```python
from build123d import *

# Parameters (mm, degrees)
F1_DEPTH = 77.5
F3_DEPTH = 15
F3_TAPER = -30
F4_W     = 9.7201652825
F4_H     = 81.3968237489
F5_DEPTH = 15


with BuildPart() as f1:
    # F0 (on Front) → F1 (new body, symmetric)
    with BuildSketch(Plane.XZ):
        Polygon((-0.1256162198, -11.1232604972), (9.5702180536, -5.6704170861), (9.6958342734, 5.4528434111), (0.1256162198, 11.1232604972), (-9.5702180536, 5.6704170861), (-9.6958342734, -5.4528434111), align=None)
    extrude(amount=F1_DEPTH, both=True)

    # F2 (on face) → F3 (join)
    with BuildSketch(Plane(origin=(0, 77.5, 0), x_dir=(-1, 0, 0), z_dir=(0, 1, 0))):
        Polygon((0.2229186467, -19.7393472), (17.2062354526, -9.676620389), (16.983316806, 10.062726811), (-0.2229186467, 19.7393472), (-17.2062354526, 9.676620389), (-16.983316806, -10.062726811), align=None)
        Polygon((9.6958342734, -5.4528434111), (0.1256162198, -11.1232604972), (-9.5702180536, -5.6704170861), (-9.6958342734, 5.4528434111), (-0.1256162198, 11.1232604972), (9.5702180536, 5.6704170861), align=None, mode=Mode.SUBTRACT)
        Polygon((-9.5702180536, -5.6704170861), (0.1256162198, -11.1232604972), (9.6958342734, -5.4528434111), (9.5702180536, 5.6704170861), (-0.1256162198, 11.1232604972), (-9.6958342734, 5.4528434111), align=None)
    extrude(amount=F3_DEPTH, taper=F3_TAPER)

    # F4 (on Top) → F5 (join)
    with BuildSketch(Plane.XY):
        with Locations((-0.1620021649, 46.2903873995)):
            Rectangle(F4_W, F4_H)
    extrude(amount=F5_DEPTH)


solid = f1.part
```
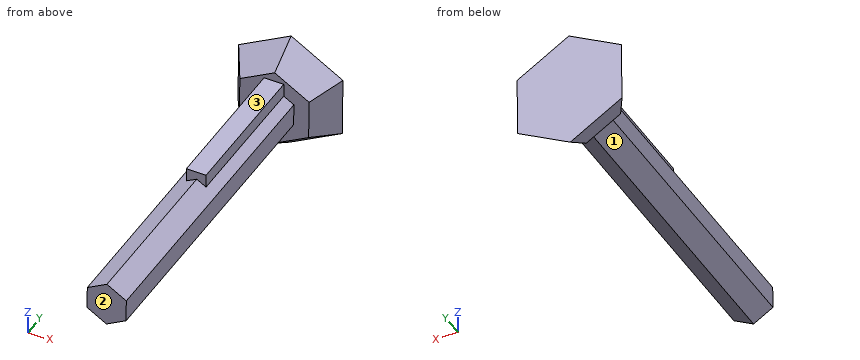
Input: part model. Units: mm. Frame: model coordinates. Face numbers are marked on the shaded views. A direction names the side the tool comes from. Coordinates: 2 decimals unless noted, no trailing zeros. Loops run counter-clockwise (first coordinate to the right, second up) from the corner with the lowest first, then second, coordinate; pieces in that order, holes last. Notation, with made-up numbers: (78, 84) - (91, 84) arc R32 cw to (91, 121) - close; hole circle Ø9 at (-24.75, 51). An arc over 180 degrees is marked (long way). Answer in a Markdown table with one row per item.
(1) Cut plane B-B on y = 2. Output: boundary loops of the cut face in (x, z).
Model answer:
| item | result |
|---|---|
| outline | (-9.7, -5.45) - (-0.13, -11.12) - (9.57, -5.67) - (9.7, 5.45) - (0.13, 11.12) - (-9.57, 5.67) - close |
(2) Material intervals for L1, parallel to Y at x = -1, z = -14.5; L2, parallel to X at y = -32.5, z = -3.5; L3, parallel to Y at x = 23, z = 6.5, sorted ascending. Write a range as from..to.
Model answer:
| item | result |
|---|---|
| L1 | y = 77.5..92.5 |
| L2 | x = -9.67..9.59 |
| L3 | y = 87.6..92.5 |
(3) Pin query (flat end, axial travel): P1, Ø8, axis at x = 1.5, y = 43.5, coming from the +Z side; P2, Ø8, axis at y = -53, z = 16.5, coming from the -X side; P3, Ø7, axis at y = 49, z = 13, coming from the +X side; P4, Ø3, axis at y = 75.5, z = -6, coming from the -X side. Return the tip coordinate at first contact, or that it passes through.
Model answer:
| item | result |
|---|---|
| P1 | stops at z = 15 |
| P2 | passes through |
| P3 | stops at x = 4.7 |
| P4 | stops at x = -9.7 |
(4) Cut plane A-A on y = 54.5. Output: boundary loops of the cut face in (x, z), plus the area to 3 significant figures.
Model answer:
| item | result |
|---|---|
| outline | (-9.7, -5.45) - (-0.13, -11.12) - (9.57, -5.67) - (9.7, 5.45) - (4.7, 8.41) - (4.7, 15) - (-5.02, 15) - (-5.02, 8.23) - (-9.57, 5.67) - close |
| area | 373 mm² |
(5) Set-up query: the marked faces 1, 2 and 3. Return all of +Z, -Z, +X, -X, +Y, -Y with unobstructed straight access to the full face (end or side cutting, diameter ignored); none if empty.
Model answer:
| item | result |
|---|---|
| face 1 | -Z, -X, -Y |
| face 2 | +Z, -Z, +X, -X, -Y |
| face 3 | +Z, +X, -X, -Y |
